Could you check a few things on this model? Use its own coordinates, in mm. A direction names the side the tool comes from. Give positions to 0.01 mm unless a question says otherwise; leave off trailing zeros. Loops run counter-clockwise (first coordinate to the right, second up) from the corner with the lowest first, then second, coordinate; pieces in that order, holes last. Notation, with made-up numbers: (-16.75, -14) -> (27.25, -14) arc R21 cw to (27.25, 3) -> close; hole circle Ø9 at (40.5, 16). An arc over 180 degrees is marked (long way). Put each result on its own line as item: value.
```python
from build123d import *

# Parameters (mm, degrees)
BOSS_EXTRUDE1_START     = -88.9
BOSS_EXTRUDE1_DEPTH     = 393.7
SKETCH3_R               = 2.4892
CUT_EXTRUDE2_DEPTH      = 1
CUT_EXTRUDE2_DEPTH_BACK = 51.8


with BuildPart() as part:
    # Sketch1 → Boss-Extrude1 (new body)
    with BuildSketch(Plane(origin=(0, 0, 0), x_dir=(-1, 0, 0), z_dir=(0, 0, -1)).offset(BOSS_EXTRUDE1_START)):
        with BuildLine():
            Line((-12.7, 25.146), (-12.7, -25.146))
            ThreePointArc((-12.7, -25.146), (-12.625605122, -25.325605122), (-12.446, -25.4))
            Line((-12.446, -25.4), (12.446, -25.4))
            ThreePointArc((12.446, -25.4), (12.625605122, -25.325605122), (12.7, -25.146))
            Line((12.7, -25.146), (12.7, 25.146))
            ThreePointArc((12.7, 25.146), (12.625605122, 25.325605122), (12.446, 25.4))
            Line((12.446, 25.4), (-12.446, 25.4))
            ThreePointArc((-12.446, 25.4), (-12.625605122, 25.325605122), (-12.7, 25.146))
        make_face()
        with BuildLine():
            Line((-11.1125, -22.225), (-11.1125, 22.225))
            ThreePointArc((-11.1125, 22.225), (-10.647532015, 23.347532015), (-9.525, 23.8125))
            Line((-9.525, 23.8125), (9.525, 23.8125))
            ThreePointArc((9.525, 23.8125), (10.647532015, 23.347532015), (11.1125, 22.225))
            Line((11.1125, 22.225), (11.1125, -22.225))
            ThreePointArc((11.1125, -22.225), (10.647532015, -23.347532015), (9.525, -23.8125))
            Line((9.525, -23.8125), (-9.525, -23.8125))
            ThreePointArc((-9.525, -23.8125), (-10.647532015, -23.347532015), (-11.1125, -22.225))
        make_face(mode=Mode.SUBTRACT)
    extrude(amount=-BOSS_EXTRUDE1_DEPTH)

    # Sketch3 → Cut-Extrude2 (cut, two sides)
    with BuildSketch(Plane.XZ.offset(25.4)) as cut_extrude2_sk:
        with Locations((0, 165.1)):
            Circle(SKETCH3_R)
        with Locations((0, 182.418181818)):
            Circle(SKETCH3_R)
        with Locations((0, 199.736363636)):
            Circle(SKETCH3_R)
        with Locations((0, 217.054545455)):
            Circle(SKETCH3_R)
        with Locations((0, 234.372727273)):
            Circle(SKETCH3_R)
        with Locations((0, 251.690909091)):
            Circle(SKETCH3_R)
        with Locations((0, 269.009090909)):
            Circle(SKETCH3_R)
        with Locations((0, 286.327272727)):
            Circle(SKETCH3_R)
        with Locations((0, 303.645454545)):
            Circle(SKETCH3_R)
        with Locations((0, 320.963636364)):
            Circle(SKETCH3_R)
        with Locations((0, 338.281818182)):
            Circle(SKETCH3_R)
        with Locations((0, 419.1)):
            Circle(SKETCH3_R)
        with Locations((0, 444.5)):
            Circle(SKETCH3_R)
        with Locations((0, 355.6)):
            Circle(SKETCH3_R)
    extrude(amount=CUT_EXTRUDE2_DEPTH, mode=Mode.SUBTRACT)
    extrude(cut_extrude2_sk.sketch, amount=-CUT_EXTRUDE2_DEPTH_BACK, mode=Mode.SUBTRACT)


solid = part.part
```
1. If we section it at A-A (y = -15.5): List the corners of the cut face in (x, z) for me.
Recorded:
outline: (-12.7, 88.9) -> (-11.11, 88.9) -> (-11.11, 482.6) -> (-12.7, 482.6) -> close; (11.11, 88.9) -> (12.7, 88.9) -> (12.7, 482.6) -> (11.11, 482.6) -> close
2. If we section it at B-B (x = -6): List the corners of the cut face in (y, z) for me, then the cut area to 3 significant figures.
Recorded:
outline: (-25.4, 88.9) -> (-23.81, 88.9) -> (-23.81, 482.6) -> (-25.4, 482.6) -> close; (23.81, 88.9) -> (25.4, 88.9) -> (25.4, 482.6) -> (23.81, 482.6) -> close
area: 1,250 mm^2
3. Thinking about a two-plate mould opening in X: for faces 1 (the face through (12.7, 0, 283)), 2 (the face through (11.3, 2, 482.6)), 3 (the face through (0, 23.812, 283)), which applies, pulls with the +X half, pulls with the -X half, needs draft (parallel to the pull), parting line crosses it, or undercut?
Recorded:
face 1: pulls with the +X half
face 2: needs draft
face 3: undercut
4. I need wall thicknesses on line 1 (Y direction, x = 5, z = 285); line 2 (X direction, y = 14.5, z = 262.5); line 3 (X direction, y = 24.35, z = 165.1). Which ranges of each line are inside material? Lowest first, please.
Recorded:
line 1: y = -25.4 to -23.81, 23.81 to 25.4
line 2: x = -12.7 to -11.11, 11.11 to 12.7
line 3: x = -12.7 to -2.49, 2.49 to 12.7
5. For faces 4 (the face through (11.112, 0, 283)), 5 (the face through (-12.7, 0, 283)), which set-ups out of +Z, -Z, +X, -X, +Y, -Y let a thin tool reach every point of the face, with its end or its side?
Recorded:
face 4: +Z, -Z
face 5: +Z, -Z, -X, +Y, -Y
